For this review, take the finished solid that the model builds, in its own axes (mm). A direction names the side the tool comes from. Coordinates: 2 decimals unless noted, no trailing zeros. Loops run counter-clockwise (first coordinate to the right, second up) from the corner with the lowest first, then second, coordinate; pieces in that order, holes last. Notation, with made-up numbers: (83.5, -30) -> (128.5, -30) arc R21 ccw to (128.5, -5) -> close; hole circle Ø1 at (-38, 35.25). An arc over 180 degrees is marked (long way). Answer in a Markdown table with one row per item.
Autodesk Inventor part; units mm, degrees
ref_plane "YZ Plane" through (0, 0, 0) normal (1, 0, 0) x (0, 1, 0)
ref_plane "XZ Plane" through (0, 0, 0) normal (0, 1, 0) x (-1, 0, 0)
ref_plane "XY Plane" through (0, 0, 0) normal (0, 0, 1) x (1, 0, 0)
sketch "Szkic2" plane through (0, 0, 0) normal (0, 1, 0) x (-1, 0, 0)
  line L0 (-12.5, 6) -> (12.5, 6)
  line L1 (12.5, 6) -> (12.5, -6)
  line L2 (12.5, -6) -> (-12.5, -6)
  line L3 (-12.5, -6) -> (-12.5, 6)
  line L4 (-12.5, 6) -> (12.5, -6) construction
  line L5 (12.5, 6) -> (-12.5, -6) construction
  line L6 (-12.5, 0) -> (-6.5, 0)
  circle A0 centre (-6.5, 0) radius 5
  line L7 (12.5, 0) -> (12.5, 2)
  line L8 (12.5, 2) -> (0.5, 2)
  line L9 (0.5, 2) -> (0.5, 6)
  line L10 (12.5, -6) -> (12.5, 6)
  line L11 (12.5, -2) -> (0.5, -2)
  line L12 (0.5, -2) -> (0.5, -6)
  point P0 (0, 0)
  point P1 (0.5, -6)
  point P2 (12.5, -2)
  dimension "d11" = 25
  dimension "d12" = 12
  dimension "d13" = 6
  dimension "d14" = 10
  dimension "d15" = 2
  dimension "d16" = 12
extrude "Wyciągnięcie proste3" add sketch "Szkic2" along normal blind 10 contours L0 L9 L8 L1 L11 L12 L2 L3
sketch "Szkic3" plane through (-12.5, 0, 2) normal (0, 0, 1) x (1, 0, 0)
  line L0 (0, 0) -> (0, 10)
  line L1 (12, 0) -> (0, 0)
  line L2 (0, 10) -> (0, 0)
  line L3 (12, 0) -> (12, 10)
  circle A0 centre (3, 5) radius 2
  point P0 (12.5, 0)
  dimension "d19" = 4
  dimension "d23" = 9
extrude "Wyciągnięcie proste4" cut sketch "Szkic3" against normal blind 32.75
fillet "Zaokrąglenie1" radius 5 6 edges at (-12.5, 0, 0) (-12.5, 10, 0) (-0.5, 0, 4) (-0.5, 10, 4) (-0.5, 0, -4) (-0.5, 10, -4)
properties part number "Knee"
Item 1: Take a section at B-B, the plane x = 6.5. State the section outline as (y, z) points.
Worked answers:
| item | result |
|---|---|
| outline | (0, -6) -> (10, -6) -> (10, -5) -> (0, -5) -> close; (0, 5) -> (10, 5) -> (10, 6) -> (0, 6) -> close |
Item 2: The part is to be moulded in two halves that separate along X. For faces 1 (the cylindrical face through (-12.5, 4.9, 0)), 2 (the flat face through (12, 0, 0)), 3 (the cylindrical face through (-9.76, 6.983, 0.028)), say which applies: +X half, -X half, draft (parallel to the pull), parting line (faces both ways), or undercut.
Worked answers:
| item | result |
|---|---|
| face 1 | -X half |
| face 2 | draft |
| face 3 | undercut |
Item 3: Take a section at A-A, the plane z = 0. State the section outline as (x, y) points.
Worked answers:
| item | result |
|---|---|
| outline | (-7.5, 0) -> (1.5, 0) -> (1.5, 10) -> (-7.5, 10) arc R5 ccw to start; (11.5, 0) -> (12.5, 0) -> (12.5, 10) -> (11.5, 10) -> close; hole circle Ø4 at (-9.5, 5) |
Item 4: Take a section at D-D, the plane y = 6. State the section outline as (x, z) points, and give its area (3 significant figures).
Worked answers:
| item | result |
|---|---|
| outline | (-12.4, -2) -> (-11.23, -2) -> (-11.23, 2) -> (-12.4, 2) -> close; (-7.77, -2) -> (-0.4, -2) -> (-0.4, -6) -> (12.5, -6) -> (12.5, 6) -> (-0.4, 6) -> (-0.4, 2) -> (-7.77, 2) -> close; hole circle Ø10 at (6.5, 0) |
| area | 110 mm² |
Item 5: For faces 4 (the cylindrical face through (-0.5, 4.9, -4)), 5 (the cylindrical face through (1.73, 4.93, -1.5)), 6 (the cylindrical face through (-0.5, 4.9, 4)), list the 3-axis set-ups (+Z, -Z, +X, -X, +Y, -Y) from which the entire face can be reached by the end or side of a thin tool; tool diameter is ignored.
Worked answers:
| item | result |
|---|---|
| face 4 | -Z, -X |
| face 5 | +Y, -Y |
| face 6 | +Z, -X |
Item 6: Take a section at C-C, the plane y = 8.25. State the section outline as (x, z) points, and give its area (3 significant figures).
Worked answers:
| item | result |
|---|---|
| outline | (-11.3, -2) -> (0.7, -2) -> (0.7, -6) -> (12.5, -6) -> (12.5, 6) -> (0.7, 6) -> (0.7, 2) -> (-11.3, 2) -> close; hole circle Ø10 at (6.5, 0) |
| area | 111 mm² |
Item 7: Insertion check: pin 1 (5 mm diameter, centred on x = -8.5, y = 4.5, fed in from -Z). The pin has a flat end and moves straight along its axis. Give the tip position at first contact, or say it passes through.
Worked answers:
| item | result |
|---|---|
| pin 1 | z = -2 |
Item 8: For L1, parallel to X at y = 4, z = 0; L2, parallel to Z at x = 6.5, y = 2; L3, parallel to X at y = 3.5, z = -1, list the stretches that pass through material, from the lowest coordinate up.
Worked answers:
| item | result |
|---|---|
| L1 | -12.4 to -11.23, -7.77 to 1.5, 11.5 to 12.5 |
| L2 | -6 to -5, 5 to 6 |
| L3 | -12.27 to -10.82, -8.18 to 1.6, 11.4 to 12.5 |
